from build123d import *

# Parameters (mm, degrees)
SKETCH1_R           = 0.3
BOSS_EXTRUDE1_DEPTH = 26
SKETCH2_W           = 1
SKETCH2_H           = 1.5


with BuildPart() as part:
    # Sketch1 → Boss-Extrude1 (new body)
    with BuildSketch(Plane.XY):
        Circle(SKETCH1_R)
    extrude(amount=BOSS_EXTRUDE1_DEPTH)

    # Sketch2 → Revolve1 (revolve)
    with BuildSketch(Plane(origin=(0, 0, 0), x_dir=(1, 0, 0), z_dir=(0, 1, 0))):
        with Locations((0.5, -5.003)):
            Rectangle(SKETCH2_W, SKETCH2_H)
        with Locations((0.5, -8.503)):
            Rectangle(SKETCH2_W, SKETCH2_H)
        with Locations((0.5, -17.01)):
            Rectangle(SKETCH2_W, SKETCH2_H)
        with Locations((0.5, -20.51)):
            Rectangle(SKETCH2_W, SKETCH2_H)
    revolve(axis=Axis((0, 0, 0), (0, 0, 1)))


solid = part.part
Here's how the part is built. I have some questions about the finished solid (model axes, mm). A direction names the side the tool comes from. Give positions to 0.01 mm unless a question says otherwise; leave off trailing zeros. Order: outer loops, then holes, each group sorted by start corner. A loop starts at its lowest first (then second) coordinate and runs counter-clockwise, first axis right, second up. Notation, with made-up numbers: M -20,47 L -13,47 A22 ccw -13,86 Z; hole C 77,-28 d1. An arc over 180 degrees is marked long. Answer as a JSON object with one key per item and string values. Group by question number.
1) Suppose I cut it at C-C, the plane z = 9. Write out the boundary of the cut face in (x, y), plus the area to 3 significant figures.
2) I'm going to push a flat-ended pin straight in: pin 1 Ø1 at (x, y) = (1, 0) entering from -Z. Where does the tip first touch, or does it pass through?
3) Suppose I cut it at A-A, the plane x = -0.55. Write out the boundary of the cut face in (y, z).
4) On a 3-axis mill with a long thin cutter (end or side, diameter ignored), from which of +Z, -Z, +X, -X, +Y, -Y can I reach the whole of each face in a straight line? I mean faces 1 (the flat face through (-0.43, -0.21, 9.253)), 2 (the cylindrical face through (0, -1, 8)). Say none if no direction works.
5) Please list where these lines run through material, in increasing order: L1, parallel to Z at x = 0.05, y = 0.45; L2, parallel to Y at x = -0.05, z = 19.5; L3, parallel to Y at x = 0.2, z = 18.5. Write a range as [from, to].
6) We'd pull the mould along Z, two halves only. Please class faces 3 (the cylindrical face through (0, -1, 5)), 4 (the flat face through (-0.43, -0.21, 21.26)), 5 (the flat face through (-0.43, -0.21, 4.253)), 6 (the flat face through (-0.43, -0.21, 19.76)): pulls with the +Z half, pulls with the -Z half, needs draft (parallel to the pull), parting line crosses it, or undercut.
7) Suppose I cut it at B-B, the plane z = 18. Write out the boundary of the cut face in (x, y), plus the area to 3 significant figures.
Results found:
{
 "1": {"outline": "C 0,0 d2", "area": "3.14 mm²"},
 "2": {"pin 1": "z = 4.25"},
 "3": {"outline": "M -0.84,4.25 L 0.84,4.25 L 0.84,5.75 L -0.84,5.75 Z; M -0.84,7.75 L 0.84,7.75 L 0.84,9.25 L -0.84,9.25 Z; M -0.84,16.26 L 0.84,16.26 L 0.84,17.76 L -0.84,17.76 Z; M -0.84,19.76 L 0.84,19.76 L 0.84,21.26 L -0.84,21.26 Z"},
 "4": {"face 1": "none", "face 2": "+Z, -Z"},
 "5": {"L1": "[4.25, 5.75], [7.75, 9.25], [16.26, 17.76], [19.76, 21.26]", "L2": "[-0.3, 0.3]", "L3": "[-0.22, 0.22]"},
 "6": {"face 3": "needs draft", "face 4": "pulls with the +Z half", "face 5": "pulls with the -Z half", "face 6": "undercut"},
 "7": {"outline": "C 0,0 d0.6", "area": "0.283 mm²"}
}
